from build123d import *

# Parameters (mm, degrees)
F0_W     = 152.4
F0_H     = 114.3
F1_DEPTH = 91.948
F3_DEPTH = 175.38727
F4_W     = 31.75
F4_H     = 114.3
F5_DEPTH = 79.248
F6_W     = 31.75
F6_H     = 114.3
F7_DEPTH = 79.248


with BuildPart() as f1:
    # F0 (on Top) → F1 (new body)
    with BuildSketch(Plane.XY):
        Rectangle(F0_W, F0_H)
    extrude(amount=F1_DEPTH)

    # F2 (on face) → F3 (cut)
    with BuildSketch(Plane.XZ.offset(57.15)):
        with BuildLine():
            Line((31.75, 91.948), (-31.75, 91.948))
            ThreePointArc((-31.75, 91.948), (0, 60.198), (31.75, 91.948))
        make_face()
    extrude(amount=-F3_DEPTH, mode=Mode.SUBTRACT)

    # F4 (on face) → F5 (cut)
    with BuildSketch(Plane.XY.offset(91.948)):
        with Locations((60.325, 0)):
            Rectangle(F4_W, F4_H)
    extrude(amount=-F5_DEPTH, mode=Mode.SUBTRACT)

    # F6 (on face) → F7 (cut)
    with BuildSketch(Plane.XY.offset(91.948)):
        with Locations((-60.325, 0)):
            Rectangle(F6_W, F6_H)
    extrude(amount=-F7_DEPTH, mode=Mode.SUBTRACT)


solid = f1.part
Read the model definition and answer for the solid it produces. Units are mm, in the model's axes. A direction names the side the tool comes from. Give positions to 0.01 mm unless a question says otherwise; leave off trailing zeros. Write each loop counter-clockwise with the first axis right and the second up, starting at its lowest first coordinate (ties: lowest second). Pieces come first, ordered by that corner, then holes. Notation, with made-up numbers: (-1.5, 35) - (55.5, 35) arc R17 cw to (55.5, 62) - close; hole circle Ø6 at (-22, -15.75). An arc over 180 degrees is marked (long way). Answer in a Markdown table with one row per item. Add a question column.
Item 1: Section D-D, the plane z = 39 is taken. Write down the section's boundary in (x, y), and give its area (3 significant figures).
Item 2: Find the intervals of material crossed by L1, parallel to Z at x = 44.5, y = 41.5; L2, parallel to X at y = -8.5, z = 42; L3, parallel to X at y = -8, z = 66.5, in increasing order.
Item 3: Section B-B, the plane y = -9 is taken. Write down the section's boundary in (x, z), and give its area (3 significant figures).
Item 4: Section C-C, the plane x = 0 is taken. Write down the section's boundary in (y, z).
Item 5: A tool of negligible diameter and unlimited length cuts with its end or side. For faces 4 (the face through (38, 1, 91.948)), 5 (the face through (44.45, -1, 53)), 6 (the face through (-61, 1, 12.7)), from which of +Z, -Z, +X, -X, +Y, -Y can it reach the whole face along a straight path? Write none if from no direction.
Item 6: Section A-A, the plane z = 70 is taken. Write down the section's boundary in (x, y), and give its area (3 significant figures).
Item 7: Determine the mould class of faces 1 (the face through (-1, -57.15, 35)), 2 (the face through (-0.698, -0.8, 60.206)), 3 (the face through (-76.2, -1, 6)) for opening direction X: pulls with the +X half, pulls with the -X half, needs draft (parallel to the pull), parting line crosses it, or undercut.
Item 8: Flat-ended cylindrical pins translate along their axes: P1, Ø8, axis at y = 6.5, z = 55, coming from the +X side; P2, Ø16, axis at x = -64.5, y = -20.5, coming from the +Z side; P3, Ø3, axis at y = -27.5, z = 41.5, coming from the -X side; P4, Ø12, axis at x = 56, z = 51, coming from the +Y side. Find the tip coordinate at first contact, or state that the pin passes through.
Recorded:
| question | item | result |
|---|---|---|
| 1 | outline | (-44.45, -57.15) - (44.45, -57.15) - (44.45, 57.15) - (-44.45, 57.15) - close |
| 1 | area | 10,200 mm2 |
| 2 | L1 | z = 0 to 12.7 |
| 2 | L2 | x = -44.45 to 44.45 |
| 2 | L3 | x = -44.45 to -18.99, 18.99 to 44.45 |
| 3 | outline | (-76.2, 0) - (76.2, 0) - (76.2, 12.7) - (44.45, 12.7) - (44.45, 91.95) - (31.75, 91.95) arc R31.75 cw to (-31.75, 91.95) - (-44.45, 91.95) - (-44.45, 12.7) - (-76.2, 12.7) - close |
| 3 | area | 7,400 mm2 |
| 4 | outline | (-57.15, 0) - (57.15, 0) - (57.15, 60.2) - (-57.15, 60.2) - close |
| 5 | face 4 | +Z, +X, -X, +Y, -Y |
| 5 | face 5 | +Z, +X, +Y, -Y |
| 5 | face 6 | +Z, -X, +Y, -Y |
| 6 | outline | (-44.45, -57.15) - (-22.94, -57.15) - (-22.94, 57.15) - (-44.45, 57.15) - close; (22.94, -57.15) - (44.45, -57.15) - (44.45, 57.15) - (22.94, 57.15) - close |
| 6 | area | 4,920 mm2 |
| 7 | face 1 | needs draft |
| 7 | face 2 | undercut |
| 7 | face 3 | pulls with the -X half |
| 8 | P1 | stops at x = 44.45 |
| 8 | P2 | stops at z = 12.7 |
| 8 | P3 | stops at x = -44.45 |
| 8 | P4 | passes through |
